For this review, take the finished solid that the model builds, in its own axes (mm). Round coordinates to 2 decimals unless told otherwise and drop trailing zeros. Order: outer loops, then holes, each group sorted by start corner. A loop starts at its lowest first (then second) coordinate and runs counter-clockwise, first axis right, second up. Notation, with made-up numbers: M 6.5,-27.5 L 62.5,-27.5 A20 ccw 62.5,9.5 Z; hole C -37.5,30.25 d9. An arc over 180 degrees is marked long. Put each result on its own line as item: value.
from build123d import *

# Parameters (mm, degrees)
SKETCH1_W           = 41.65
SKETCH1_H           = 154.2
BOSS_EXTRUDE1_DEPTH = 1.65
SKETCH3_W           = 38.35
SKETCH3_H           = 1.65
CUT_EXTRUDE1_DEPTH  = 1.65


with BuildPart() as part:
    # Sketch1 → Boss-Extrude1 (new body)
    with BuildSketch(Plane.XY):
        Rectangle(SKETCH1_W, SKETCH1_H)
    extrude(amount=BOSS_EXTRUDE1_DEPTH)

    # Sketch3 → Cut-Extrude1 (cut)
    with BuildSketch(Plane(origin=(0, 77.1, 0), x_dir=(1, 0, 0), z_dir=(0, 1, 0))):
        with Locations((0, -0.825)):
            Rectangle(SKETCH3_W, SKETCH3_H)
    cut_extrude1 = extrude(amount=-CUT_EXTRUDE1_DEPTH, mode=Mode.SUBTRACT)

    # Mirror1: Cut-Extrude1 across plane
    add(cut_extrude1.mirror(Plane.ZX), mode=Mode.SUBTRACT)


solid = part.part
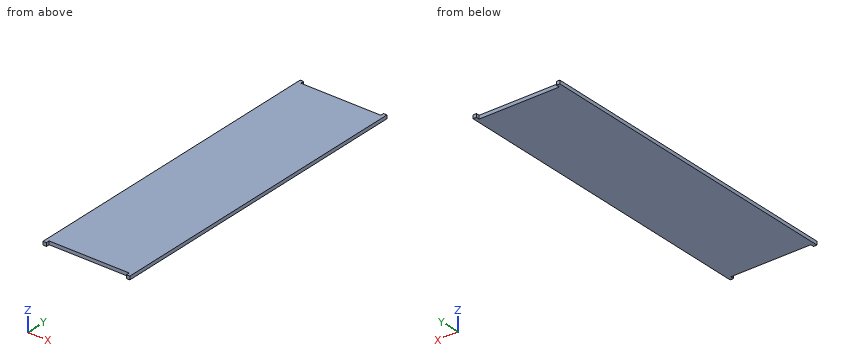
(1) Add section A-A on z = 0.7. Give the boundary of the cut face in (x, y) (3 decimals).
A:
outline: M -20.825,-77.1 L -19.175,-77.1 L -19.175,-75.45 L 19.175,-75.45 L 19.175,-77.1 L 20.825,-77.1 L 20.825,77.1 L 19.175,77.1 L 19.175,75.45 L -19.175,75.45 L -19.175,77.1 L -20.825,77.1 Z
(2) Add section B-B on x = -5.5. Give the boundary of the cut face in (y, z), then the cut area to 3 significant figures.
A:
outline: M -75.45,0 L 75.45,0 L 75.45,1.65 L -75.45,1.65 Z
area: 249 mm2
(3) Insertion check: pin 1 Ø0.8 at (x, z) = (2.5, 1) entering from -Y; pin 2 Ø0.5 at (x, z) = (2.5, 1) entering from +Y. Each pin has a flat end and moves straight along its axis. Give the tip position at first contact, or say it passes through.
A:
pin 1: stops at y = -75.45
pin 2: stops at y = 75.45
(4) To check wall thickness, follow L1, parallel to Y at x = -16, z = 0.25. State the ranges of the line that lie inside material, in increasing order.
A:
L1: y = -75.45 to 75.45
